from build123d import *

# Parameters (mm, degrees)
SKETCH2_W                = 463
SKETCH2_H                = 506
BASE_FLANGE1_DEPTH       = 1.51892
SKETCH13_R               = 1.5
SKETCH13_R_2             = 5
CUT_EXTRUDE1_DEPTH       = 1.51892
M3_CLEARANCE_HOLE2_D     = 3.6
M3_CLEARANCE_HOLE2_DEPTH = 11.938
M3_CLEARANCE_HOLE2_TIP   = 1.081549114


# Sheet-metal steps are written as plain solids
with BuildPart() as part:
    # Sketch2 → Base-Flange1 (new body)
    with BuildSketch(Plane.XY):
        with Locations((0, -15.3575)):
            Rectangle(SKETCH2_W, SKETCH2_H)
    extrude(amount=-BASE_FLANGE1_DEPTH)

    # Sketch13 → Cut-Extrude1 (cut)
    with BuildSketch(Plane(origin=(0, 0, -1.51892), x_dir=(-1, 0, 0), z_dir=(0, 0, -1))):
        with BuildLine():
            Line((156.5, 187.5), (-156.5, 187.5))
            ThreePointArc((-156.5, 187.5), (-174.17766953, 180.17766953), (-181.5, 162.5))
            Line((-181.5, 162.5), (-181.5, -162.5))
            ThreePointArc((-181.5, -162.5), (-174.17766953, -180.17766953), (-156.5, -187.5))
            Line((-156.5, -187.5), (156.5, -187.5))
            ThreePointArc((156.5, -187.5), (174.17766953, -180.17766953), (181.5, -162.5))
            Line((181.5, -162.5), (181.5, 162.5))
            ThreePointArc((181.5, 162.5), (174.17766953, 180.17766953), (156.5, 187.5))
        make_face()
        with BuildLine():
            Line((217.65, -260.115), (195.35, -260.115))
            ThreePointArc((195.35, -260.115), (193.582233047, -259.382766953), (192.85, -257.615))
            Line((192.85, -257.615), (192.85, -231.315))
            ThreePointArc((192.85, -231.315), (193.582233047, -229.547233047), (195.35, -228.815))
            Line((195.35, -228.815), (217.65, -228.815))
            ThreePointArc((217.65, -228.815), (219.417766953, -229.547233047), (220.15, -231.315))
            Line((220.15, -231.315), (220.15, -257.615))
            ThreePointArc((220.15, -257.615), (219.417766953, -259.382766953), (217.65, -260.115))
        make_face()
        with BuildLine():
            Line((156.5, -243.3575), (-156.5, -243.3575))
            ThreePointArc((-156.5, -243.3575), (-173.510345436, -250.03679728), (-181.431318552, -266.505648148))
            ThreePointArc((-181.431318552, -266.505648148), (-182.064996401, -267.823156218), (-183.425824036, -268.3575))
            Line((-183.425824036, -268.3575), (183.425824036, -268.3575))
            ThreePointArc((183.425824036, -268.3575), (182.064996401, -267.823156218), (181.431318552, -266.505648148))
            ThreePointArc((181.431318552, -266.505648148), (173.510345436, -250.03679728), (156.5, -243.3575))
        make_face()
        with Locations((188.5, -244.465)):
            Circle(SKETCH13_R)
        with BuildLine():
            Line((217, -207.715), (217, -218.715))
            ThreePointArc((217, -218.715), (216.414213562, -220.129213562), (215, -220.715))
            Line((215, -220.715), (204, -220.715))
            ThreePointArc((204, -220.715), (202.585786438, -220.129213562), (202, -218.715))
            Line((202, -218.715), (202, -207.715))
            ThreePointArc((202, -207.715), (202.585786438, -206.300786438), (204, -205.715))
            Line((204, -205.715), (215, -205.715))
            ThreePointArc((215, -205.715), (216.414213562, -206.300786438), (217, -207.715))
        make_face()
        with Locations((193.6, -215.215)):
            Circle(SKETCH13_R_2)
    extrude(amount=-CUT_EXTRUDE1_DEPTH, mode=Mode.SUBTRACT)

    # M3 Clearance Hole2
    with Locations(Plane.XY):
        with Locations((217.8375, -129.361666667), (217.8375, -57.560833333), (217.8375, 14.24), (217.8375, 86.040833333), (217.8375, 157.841666667), (-217.8375, 157.841666667), (-217.8375, 86.040833333), (-217.8375, 14.24), (-217.8375, -57.560833333), (-217.8375, -129.361666667), (-145.225, -201.1625), (-72.6125, -201.1625), (0, -201.1625), (72.6125, -201.1625), (145.225, -201.1625), (-217.8375, 229.6425), (217.8375, 229.6425), (217.8375, -201.1625), (-217.8375, -201.1625)):
            Hole(M3_CLEARANCE_HOLE2_D / 2, depth=M3_CLEARANCE_HOLE2_DEPTH)
            with Locations((0, 0, -(M3_CLEARANCE_HOLE2_DEPTH + M3_CLEARANCE_HOLE2_TIP / 2))):  # 118° drill point
                Cone(0, M3_CLEARANCE_HOLE2_D / 2, M3_CLEARANCE_HOLE2_TIP, mode=Mode.SUBTRACT)


solid = part.part
The model under review builds one solid part; all positions refer to its coordinate system, in mm. A direction names the side the tool comes from. Round coordinates to 2 decimals unless told otherwise and drop trailing zeros. Order: outer loops, then holes, each group sorted by start corner. A loop starts at its lowest first (then second) coordinate and runs counter-clockwise, first axis right, second up. Notation, with made-up numbers: (3, 77.25) -> (7, 77.25) arc R21 ccw to (7, 98.25) -> close; hole circle Ø7 at (41, 23). An arc over 180 degrees is marked (long way). Write item = value, one per line. Start each with the question number.
Item 1: Consider section C-C on z = -0.85. Count the separate pieces of the cut face and the enclosed holes in it, plus the area to 3 significant figures.
Item 2: For faces 1 (the face through (203, -12, -1.519)), 2 (the face through (-173.701, -250.216, -0.77)), 3 (the face through (173.982, 180.371, -0.77)), list the 3-axis set-ups (+Z, -Z, +X, -X, +Y, -Y) from which the entire face can be reached by the end or side of a thin tool; tool diameter is ignored.
Item 3: For line 1 along X through (y, z) = (-57, -0.2); line 2 along X through (y, z) = (-51.5, -0.1); line 3 along Y through (x, z) = (-130.5, -1.3), list the stretches that pass through material, from the lowest coordinate up.
Item 4: Consider section A-A on y = -101. Write out the cut boundary in (x, z).
Item 5: Mouldability with a two-part tool opening along Y and no side actions: class faces 4 (the face through (203, -12, 0)), 5 (the face through (-173.982, -180.371, -0.77)), 6 (the face through (173.32, -249.86, -0.77)) as released by +Y, released by -Y, zero draft, split by the parting line, or undercut.
Item 6: Consider section B-B on x = 121. Write out the cut boundary in (y, z).
Conclusion:
q1.separate_pieces = 1
q1.enclosed_holes = 24
q1.area = 88,500 mm2
q2.face_1 = -Z, +X, -X, +Y, -Y
q2.face_2 = +Z, -Z, -Y
q2.face_3 = +Z, -Z
q3.line_1 = -231.5 to -219.55, -216.13 to -181.5, 181.5 to 216.13, 219.55 to 231.5
q3.line_2 = -231.5 to -181.5, 181.5 to 231.5
q3.line_3 = -243.36 to -187.5, 187.5 to 237.64
q4.outline = (-231.5, -1.52) -> (-181.5, -1.52) -> (-181.5, 0) -> (-231.5, 0) -> close; (181.5, -1.52) -> (231.5, -1.52) -> (231.5, 0) -> (181.5, 0) -> close
q5.face_4 = zero draft
q5.face_5 = undercut
q5.face_6 = released by -Y
q6.outline = (-243.36, -1.52) -> (-187.5, -1.52) -> (-187.5, 0) -> (-243.36, 0) -> close; (187.5, -1.52) -> (237.64, -1.52) -> (237.64, 0) -> (187.5, 0) -> close
